Build history of the part. All positions in model axes, mm. A direction names the side the tool comes from. Give positions to 0.01 mm unless a question says otherwise; leave off trailing zeros. Loops run counter-clockwise (first coordinate to the right, second up) from the corner with the lowest first, then second, coordinate; pieces in that order, holes last.
1) Flat gauge pins, fed straight in: P1, Ø1, axis at x = 6, y = -8, coming from the +Z side; P2, Ø3, axis at x = 7.5, z = 27, coming from the +Y side; P3, Ø3.5, axis at y = -4, z = -13.8, coming from the +X side; P4, Ø3, axis at x = 7, z = -9.5, coming from the -Y side. Where does each tip first touch, or does it go through?
2) Band-saw the part on B-B on x = 3.25. State how many separate pieces and enclosed holes the cut face has, then the cut area to 3 significant figures.
3) Wall check: line 1 (Z direction, x = 8.75, y = -27); line 2 (Y direction, x = 3.25, z = -11); line 3 (Z direction, x = 6.25, y = -4.5). Give the ranges that are in metal, low to high.
4) Band-saw the part on A-A on y = -33. List the corners of the cut face in (x, z).
5) 3-axis set-ups, long thin cutter, end or side, ignore diameter. For faces 1 (the cylindrical face through (5.07, -6.141, -81.597)), 2 (the flat face through (7.471, -32, 60)), 3 (the flat face through (5, -5, 33)), 4 (the flat face through (5, -26, -72.8)), 5 (the cylindrical face through (4.93, -39.997, 63.859)): which of +Z, -Z, +X, -X, +Y, -Y reach the whole face in a straight line?
6) Band-saw the part on D-D on z = -38.5. List the corners of the cut face in (x, y), then the cut area to 3 significant figures.
7) Band-saw the part on C-C on y = -25.5. List the corners of the cut face in (x, z), then the cut area to 3 significant figures.
```python
from build123d import *

# Parameters (mm, degrees)
BOSS_EXTRUDE1_DEPTH = 10
SKETCH3_R           = 2.055
CUT_EXTRUDE1_DEPTH  = 85.739837149
SKETCH5_W           = 10
SKETCH5_H           = 13.8
BOSS_EXTRUDE2_DEPTH = 10
SKETCH10_W          = 10
SKETCH10_H          = 7.4
BOSS_EXTRUDE5_DEPTH = 2.52893219
SKETCH11_W          = 10
SKETCH11_H          = 5
BOSS_EXTRUDE6_DEPTH = 10
FILLET1_R           = 4
FILLET2_R           = 4
FILLET3_R           = 4


with BuildPart() as part:
    # Sketch1 → Boss-Extrude1 (new body)
    with BuildSketch(Plane(origin=(0, 0, 0), x_dir=(0, 0, -1), z_dir=(1, 0, 0))):
        Polygon((17.8, -5), (82.8, -5), (82.8, -15), (-65, -15), (-65, -5), (0, -5), (0, 0), (17.8, 0), align=None)
    extrude(amount=BOSS_EXTRUDE1_DEPTH)

    # Sketch3 → Cut-Extrude1 (cut, through all)
    with BuildSketch(Plane(origin=(10, 0, 0), x_dir=(0, 0, -1), z_dir=(1, 0, 0))):
        with Locations((4, -4)):
            Circle(SKETCH3_R)
        with Locations((13.8, -4)):
            Circle(SKETCH3_R)
    extrude(amount=-CUT_EXTRUDE1_DEPTH, mode=Mode.SUBTRACT)

    # Sketch5 → Boss-Extrude2 (add)
    with BuildSketch(Plane(origin=(10, 0, 0), x_dir=(0, 0, -1), z_dir=(1, 0, 0))):
        with Locations((-60, -21.9)):
            Rectangle(SKETCH5_W, SKETCH5_H)
        with Locations((77.8, -21.9)):
            Rectangle(SKETCH5_W, SKETCH5_H)
    extrude(amount=-BOSS_EXTRUDE2_DEPTH)

    # Sketch10 → Boss-Extrude5 (add)
    with BuildSketch(Plane(origin=(10, 0, 0), x_dir=(0, 0, -1), z_dir=(1, 0, 0))):
        with Locations((-60, -32.5)):
            Rectangle(SKETCH10_W, SKETCH10_H)
    boss_extrude5 = extrude(amount=-BOSS_EXTRUDE5_DEPTH)

    # Sketch11 → Boss-Extrude6 (add)
    with BuildSketch(Plane(origin=(10, 0, 0), x_dir=(0, 0, -1), z_dir=(1, 0, 0))):
        with Locations((-60, -38.7)):
            Rectangle(SKETCH11_W, SKETCH11_H)
    boss_extrude6 = extrude(amount=-BOSS_EXTRUDE6_DEPTH)

    # Mirror1: Boss-Extrude5, Boss-Extrude6 across plane
    add(boss_extrude5.mirror(Plane.XY.offset(-8.9)))
    add(boss_extrude6.mirror(Plane.XY.offset(-8.9)))

    # Fillet1
    fillet1_edges = [part.edges().sort_by_distance(p)[0] for p in [
        (5, 0, 0),
        (5, 0, -17.8),
    ]]
    fillet(fillet1_edges, radius=FILLET1_R)

    # Fillet2
    fillet2_edges = [part.edges().sort_by_distance(p)[0] for p in [
        (5, -5, -82.8),
        (5, -5, 65),
        (5, -15, 55),
        (5, -15, -72.8),
        (5, -41.2, 55),
        (5, -41.2, 65),
        (5, -41.2, -82.8),
        (5, -41.2, -72.8),
    ]]
    fillet(fillet2_edges, radius=FILLET2_R)

    # Fillet3
    fillet3_edges = [part.edges().sort_by_distance(p)[0] for p in [
        (5, -5, -17.8),
        (5, -5, 0),
    ]]
    fillet(fillet3_edges, radius=FILLET3_R)


solid = part.part
```
Findings below:
1. P1: stops at z = 64.97
1. P2: stops at y = -5
1. P3: passes through
1. P4: stops at y = -15
2. separate pieces: 3
2. enclosed holes: 2
2. area: 1,900 mm2
3. line 1: z = -82.8 to -72.8, 55 to 65
3. line 2: y = -15 to 0
3. line 3: z = -19.28 to -15.79, -11.81 to -5.99, -2.01 to 1.48
4. outline: (7.47, -82.8) - (10, -82.8) - (10, -72.8) - (7.47, -72.8) - close; (7.47, 55) - (10, 55) - (10, 65) - (7.47, 65) - close
5. face 1: -Z, +X, -X, +Y
5. face 2: +Z, -Z, -X
5. face 3: +Z, +X, -X, +Y
5. face 4: +X, -X, -Y
5. face 5: +Z, +X, -X, -Y
6. outline: (0, -15) - (10, -15) - (10, -5) - (0, -5) - close
6. area: 100 mm2
7. outline: (0, -82.8) - (10, -82.8) - (10, -72.8) - (0, -72.8) - close; (0, 55) - (10, 55) - (10, 65) - (0, 65) - close
7. area: 200 mm2
